For this review, use the dimensioned drawing (mm, ordinates from the lowest corner) and the shaded views. Coordinates: 2 decimals unless noted, no trailing zeros. Order: outer loops, then holes, each group sorted by start corner. A loop starts at its lowest first (then second) coordinate and runs counter-clockwise, first axis right, second up. Notation, with made-up numbers: (-35.75, -0.75) -> (2.25, -0.75) arc R9 ccw to (2.25, 8.25) -> close; hole circle Ø1 at (70, -18.5). An arc over 180 degrees is marked (long way). Return JSON: item names as keys, results as strings. Group by question number.
Item 1: For line 1 along Z through (x, y) = (11.75, 1.45) (1 decimal); line 2 along X through (y, z) = (1.6, 38) (1 decimal); line 3 along Z through (x, y) = (10.5, 0.8) (1 decimal), list the stretches that pass through material, from the lowest coordinate up.
Item 2: Take a section at A-A (z = 76.2). Write out the cut boundary in (x, y) (1 decimal).
Item 3: Insertion check: pin 1 (1 mm diameter, centred on y = 2, z = 25, fed in from -X) (1 decimal). The pin has a flat end and moves straight along its axis. Give the tip position at first contact, or say it passes through.
Item 4: Take a section at B-B (y = 2.6). Write out the cut boundary in (x, z) (1 decimal), then the cut area to 3 significant figures.
Item 5: Take a section at C-C (z = 13). Write out the cut boundary in (x, y) (1 decimal), then the cut area to 3 significant figures.
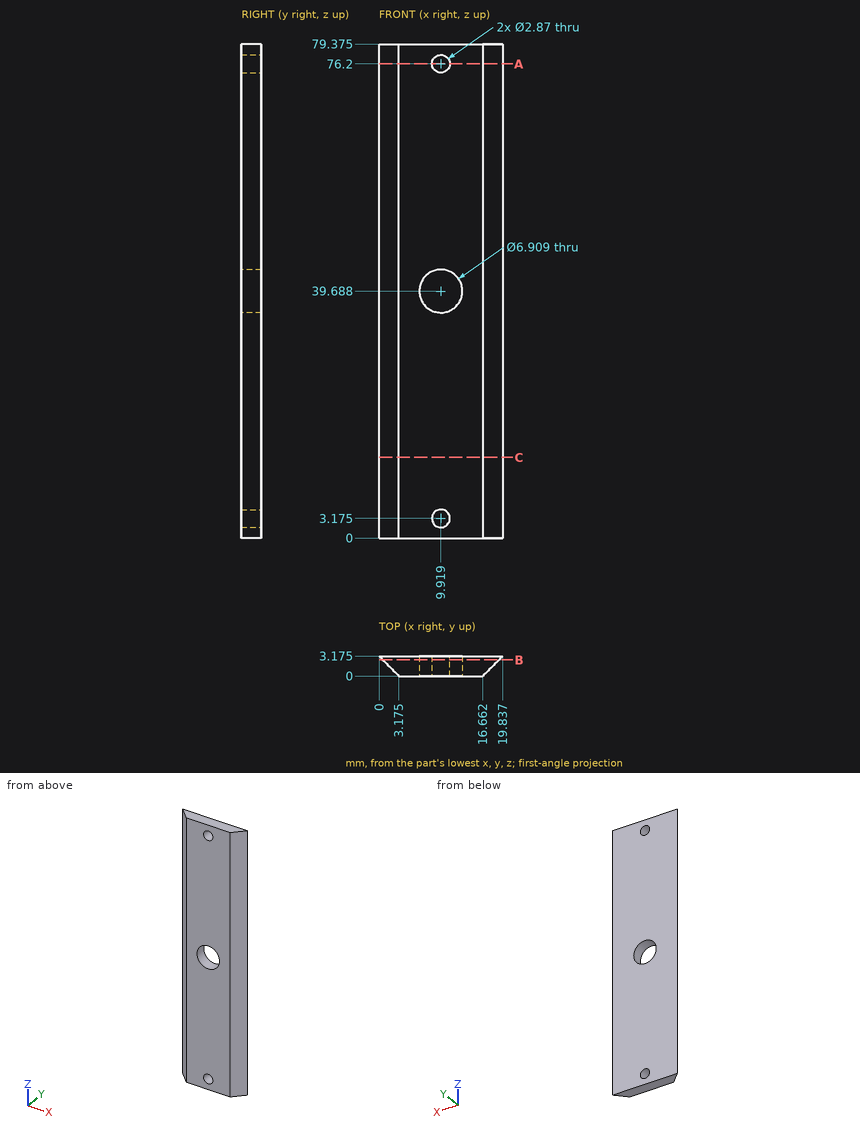
Findings below:
{
 "1": {"line 1": "z = 0 to 36.8, 42.6 to 79.4", "line 2": "x = 1.6 to 6.9, 12.9 to 18.3", "line 3": "z = 0 to 1.9, 4.5 to 36.3, 43.1 to 74.9, 77.5 to 79.4"},
 "2": {"outline": "(0, 3.2) -> (3.2, 0) -> (8.5, 0) -> (8.5, 3.2) -> close; (11.4, 0) -> (16.7, 0) -> (19.8, 3.2) -> (11.4, 3.2) -> close"},
 "3": {"pin 1": "stops at x = 0.7"},
 "4": {"outline": "(0.6, 0) -> (19.3, 0) -> (19.3, 79.4) -> (0.6, 79.4) -> close; hole circle Ø6.9 at (9.9, 39.7); hole circle Ø2.9 at (9.9, 3.2); hole circle Ø2.9 at (9.9, 76.2)", "area": "1,430 mm2"},
 "5": {"outline": "(0, 3.2) -> (3.2, 0) -> (16.7, 0) -> (19.8, 3.2) -> close", "area": "52.9 mm2"}
}
